Study the drawing (mm; zero at the part's minimum x, y, z) and answer. A direction names the side the tool comes from. Coordinates: 2 decimals unless noted, no trailing zeros. Order: outer loops, then holes, each group sorted by start corner. A loop starts at its lowest first (then second) coordinate and runs counter-clockwise, first axis right, second up. Notation, with made-up numbers: M 19.25,26.25 L 67.25,26.25 A22 ccw 67.25,62.25 Z; hole C -5.5,17 d1. An arc over 180 degrees is marked long. Use a Markdown table: item, result. Add a question column.
1) Find section B-B on z = 11.5. Write down the section's boundary in (x, y).
2) The mould has two halves that part along Y. Classify the marked faces 4, 5 and 6: released by +Y, released by -Y, zero draft, split by the parting line, or undercut.
3) Each of these flat-tipped pins is pushed along its axis until it touches: pin 1 Ø5 at (x, y) = (15, 5) entering from +Z; pin 2 Ø3.5 at (x, y) = (15, 65.4) entering from +Z; pin 3 Ø4 at (x, y) = (15.5, 20.5) entering from -Z. Where does it stop, or does it pass through?
4) For the marked faces 1, 2 and 3, determine the directions among +Z, -Z, +X, -X, +Y, -Y from which every point of the face is accessible in a straight line to the end or side of a thin tool.
5) Find section D-D on x = 2.5. Write down the section's boundary in (y, z), plus the area to 3 significant figures.
6) Find section A-A on x = 15. Write down the section's boundary in (y, z).
7) Find the intervals of material crossed by probe 1 along X at (y, z) = (65.4, 5.25); probe 2 along Y at (x, z) = (19.75, 1.5); probe 3 along Z at (x, y) = (20, 26), in increasing order. Write a range as [from, to].
8) Find section C-C on y = 66.5. Write down the section's boundary in (x, z).
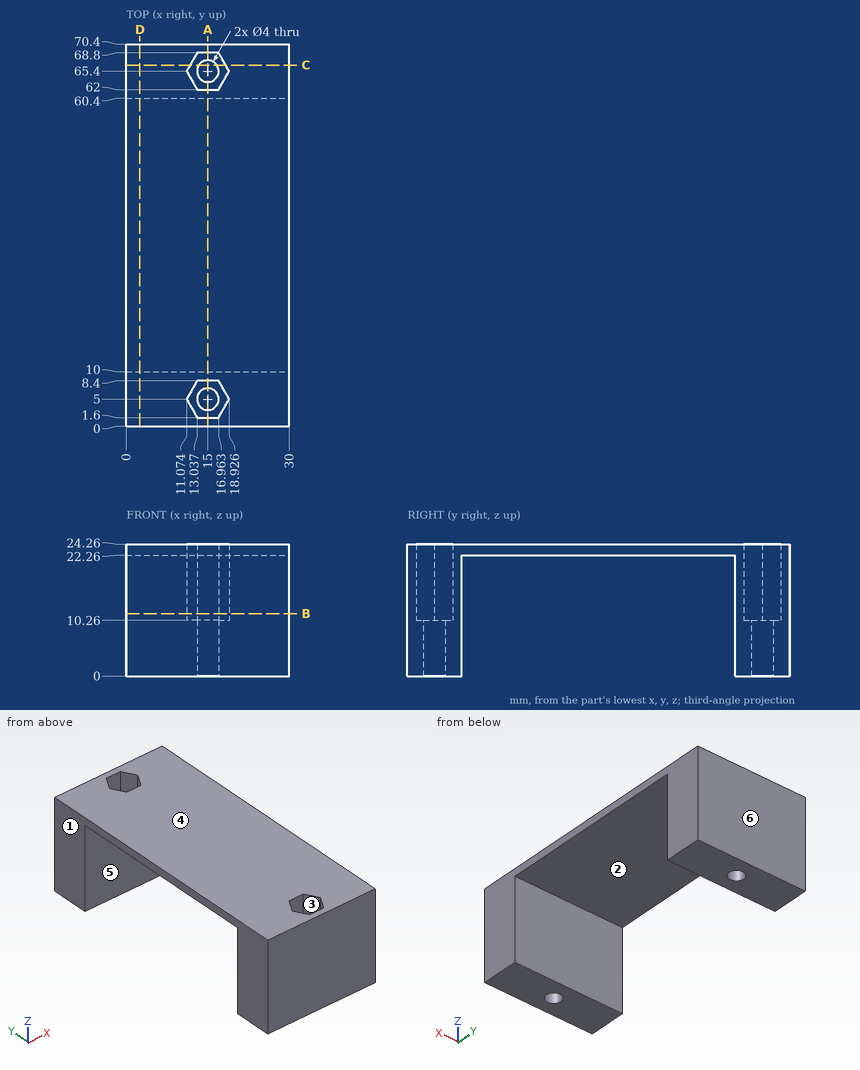
Check result:
| question | item | result |
|---|---|---|
| 1 | outline | M 0,0 L 30,0 L 30,10 L 0,10 Z; M 0,60.4 L 30,60.4 L 30,70.4 L 0,70.4 Z; hole M 11.07,5 L 13.04,1.6 L 16.96,1.6 L 18.93,5 L 16.96,8.4 L 13.04,8.4 Z; hole M 11.07,65.4 L 13.04,62 L 16.96,62 L 18.93,65.4 L 16.96,68.8 L 13.04,68.8 Z |
| 2 | face 4 | zero draft |
| 2 | face 5 | undercut |
| 2 | face 6 | released by +Y |
| 3 | pin 1 | stops at z = 10.26 |
| 3 | pin 2 | passes through |
| 3 | pin 3 | stops at z = 22.26 |
| 4 | face 1 | +Z, -Z, -X, +Y, -Y |
| 4 | face 2 | -Z, +X, -X |
| 4 | face 3 | +Z |
| 5 | outline | M 0,0 L 10,0 L 10,22.26 L 60.4,22.26 L 60.4,0 L 70.4,0 L 70.4,24.26 L 0,24.26 Z |
| 5 | area | 586 mm2 |
| 6 | outline | M 0,0 L 3,0 L 3,10.26 L 1.6,10.26 L 1.6,24.26 L 0,24.26 Z; M 7,0 L 10,0 L 10,22.26 L 60.4,22.26 L 60.4,0 L 63.4,0 L 63.4,10.26 L 62,10.26 L 62,24.26 L 8.4,24.26 L 8.4,10.26 L 7,10.26 Z; M 67.4,0 L 70.4,0 L 70.4,24.26 L 68.8,24.26 L 68.8,10.26 L 67.4,10.26 Z |
| 7 | probe 1 | x = [0, 13], [17, 30] |
| 7 | probe 2 | y = [0, 10], [60.4, 70.4] |
| 7 | probe 3 | z = [22.26, 24.26] |
| 8 | outline | M 0,0 L 13.33,0 L 13.33,10.26 L 11.71,10.26 L 11.71,24.26 L 0,24.26 Z; M 16.67,0 L 30,0 L 30,24.26 L 18.29,24.26 L 18.29,10.26 L 16.67,10.26 Z |
